```python
from build123d import *

# Parameters (mm, degrees)
F0_R     = 6.672459
F0_R_2   = 4.451297
F1_DEPTH = 25
F3_DEPTH = 12.25


with BuildPart() as f1:
    # F0 (on Front) → F1 (new body)
    with BuildSketch(Plane.XZ):
        with BuildLine():
            Line((53.057076, 8), (-16.338237, 8))
            ThreePointArc((-16.338237, 8), (-38.442924, 0), (-16.338237, -8))
            Line((-16.338237, -8), (53.057076, -8))
            ThreePointArc((53.057076, -8), (69.057076, 0), (53.057076, 8))
        make_face()
        with Locations((-25.942924, 0)):
            Circle(F0_R, mode=Mode.SUBTRACT)
        with Locations((59.057076, 0)):
            Circle(F0_R_2, mode=Mode.SUBTRACT)
    extrude(amount=F1_DEPTH)

    # F2 (on Top) → F3 (intersect, symmetric)
    with BuildSketch(Plane.XY):
        Polygon((-11.041536, -9), (-38.442924, -9), (-38.442924, -17), (-10.341627, -17), (40.699909, -8), (69.057076, -8), (69.057076, 0), (40, 0), align=None)
    extrude(amount=F3_DEPTH, both=True, mode=Mode.INTERSECT)


solid = f1.part
```
CAD build for the part. Positions are in the model's coordinates, mm. A direction names the side the tool comes from. Round coordinates to 2 decimals unless told otherwise and drop trailing zeros. Write each loop counter-clockwise with the first axis right and the second up, starting at its lowest first coordinate (ties: lowest second). Pieces come first, ordered by that corner, then holes. Notation, with made-up numbers: M -16.5,86 L 6.5,86 A31 ccw 6.5,123 Z; hole C 59.25,54.5 d8. An arc over 180 degrees is marked long. One line per question, with ' | ' between items.
1. Cut at B-B on y = -15.5. Write the cut outline in (x, z).
Working result:
outline: M -28.43,-12.25 L -23.46,-12.25 A12.5 ccw -16.34,-8 L -1.83,-8 L -1.83,8 L -16.34,8 A12.5 ccw -23.46,12.25 L -28.43,12.25 A12.5 ccw Z; hole C -25.94,0 d13.34
2. Pin check, flat tips, straight feed: pin 1 Ø6 at (x, y) = (-22.5, -15) entering from -Z; pin 2 Ø12.5 at (x, z) = (-29, 0) entering from +Y; pin 3 Ø8 at (x, y) = (-7, -8) entering from -Z; pin 4 Ø4 at (x, z) = (8, 7) entering from +Y. Stop position of each tip, or through.
Working result:
pin 1: z = -12.25 | pin 2: y = -9 | pin 3: z = -8 | pin 4: y = -5.29
3. Mould opens along Z. For faces 6 (the cylindrical face through (69.052, -3.944, -0.31)), 7 (the flat face through (19, -8, 8)), 8 (the cylindrical face through (54.61, -3.94, 0.2)) say: pulls with the +Z half, pulls with the -Z half, needs draft (parallel to the pull), parting line crosses it, or undercut.
Working result:
face 6: parting line crosses it | face 7: pulls with the +Z half | face 8: undercut
4. Cut at A-A on z = 0. Write the cut outline in (x, y).
Working result:
outline: M -38.44,-17 L -32.62,-17 L -32.62,-9 L -38.44,-9 Z; M -19.27,-17 L -10.34,-17 L 40.7,-8 L 54.61,-8 L 54.61,0 L 40,0 L -11.04,-9 L -19.27,-9 Z; M 63.51,-8 L 69.06,-8 L 69.06,0 L 63.51,0 Z
5. Which spindle directions (+Z, -Z, +X, -X, +Y, -Y) get a long thin tool onto all of the face, cutting with end or side? Do faces 1 (the flat face through (-18, -9, 0)), 2 (the flat face through (-26, -13, 12.25)), 3 (the flat face through (18, -8, -8)), 4 (the flat face through (54, 0, 0)), 5 (the flat face through (54.7, -8, -2.1)). Say none if no direction does.
Working result:
face 1: +Z, -Z, -X, +Y | face 2: +Z, +X, -X, +Y, -Y | face 3: -Z, +Y, -Y | face 4: +Z, -Z, +X, -X, +Y | face 5: +Z, -Z, +X, -Y
6. Cut at C-C on z = -5.75. Write the cut outline in (x, y).
Working result:
outline: M -37.04,-17 L -29.33,-17 L -29.33,-9 L -37.04,-9 Z; M -22.56,-17 L -10.34,-17 L 40.7,-8 L 67.24,-8 L 67.24,0 L 40,0 L -11.04,-9 L -22.56,-9 Z
7. Cut at D-D on x = -29.5. Write the cut outline in (y, z), and give its area (3 significant figures).
Working result:
outline: M -17,-11.98 L -9,-11.98 L -9,-5.65 L -17,-5.65 Z; M -17,5.65 L -9,5.65 L -9,11.98 L -17,11.98 Z | area: 101 mm2
8. Probe L1, parallel to Z at x = 36.5, y = -4.75; L2, parallel to Y at x = 52, z = 4; L3, parallel to Y at x = -17, z = 3.25. List the from-to ranges inside material, lowest first. Write a range as from..to.
Working result:
L1: -8..8 | L2: -8..0 | L3: -17..-9
